Check sheet for the drawn part. Datum: minimum x, y, z corner. Units: mm. Give positions to 0.01 mm unless a question says otherwise; leave off trailing zeros. Order: outer loops, then holes, each group sorted by start corner. A loop starts at its lowest first (then second) coordinate and runs counter-clockwise, first axis right, second up. Notation, with made-up numbers: (79, -30.75) -> (87, -30.75) arc R16 ccw to (87, -19.75) -> close; hole circle Ø7 at (31.5, 13.5). An arc over 180 degrees is marked (long way). One line per question, with ' | ' between items. Start each with the question number.
Q1. Section check B-B on x = 11.75. Record the cut outline in (y, z), plus the area to 3 significant figures.
Q2. Section check A-A on y = 258.5. Record the cut outline in (x, z).
Q3. Material ranges on probe 1 along Z at (x, y) = (16, 109); probe 2 along Y at (x, z) = (17.75, 25); probe 3 along Y at (x, z) = (10.25, 24.5), recorded low to high. Write a range as [from, to].
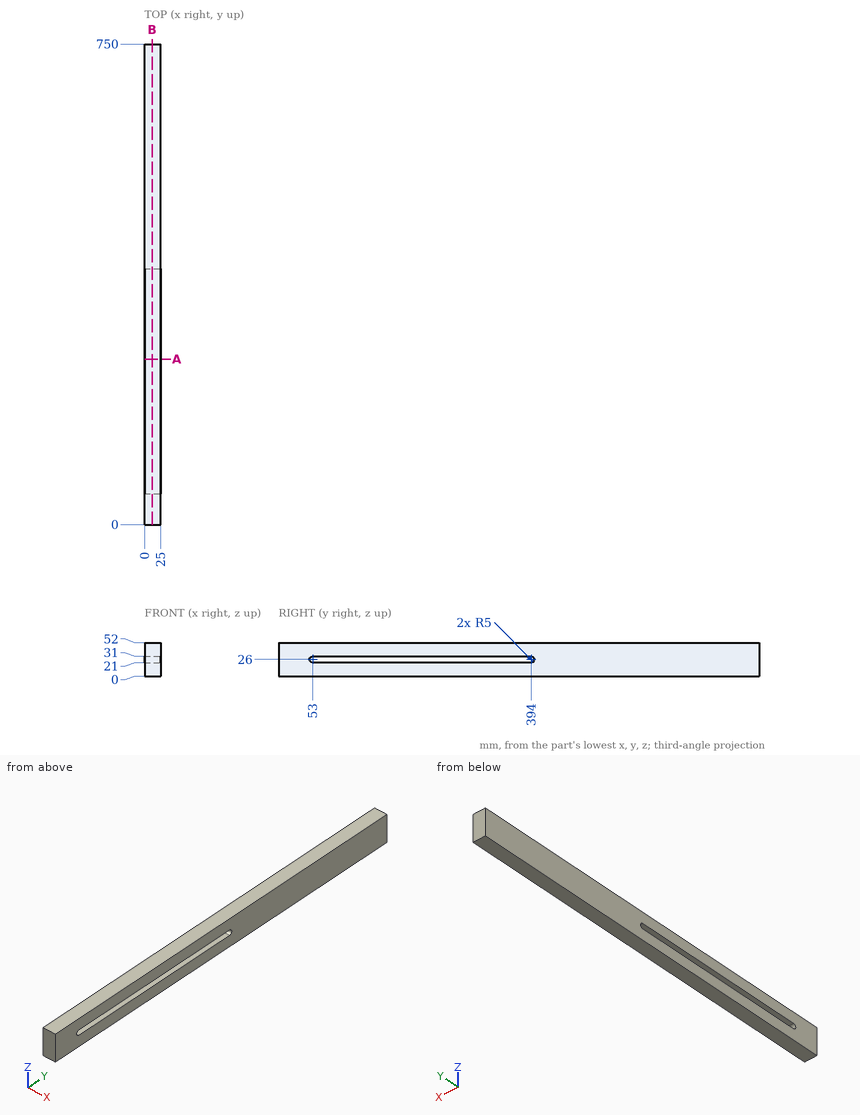
Filled in:
1) outline: (0, 0) -> (750, 0) -> (750, 52) -> (0, 52) -> close; hole (53, 21) -> (394, 21) arc R5 ccw to (394, 31) -> (53, 31) arc R5 ccw to start | area: 35,500 mm²
2) outline: (0, 0) -> (25, 0) -> (25, 21) -> (0, 21) -> close; (0, 31) -> (25, 31) -> (25, 52) -> (0, 52) -> close
3) probe 1: [0, 21], [31, 52] | probe 2: [0, 48.1], [398.9, 750] | probe 3: [0, 48.23], [398.77, 750]
